Can you work these out from the model? Positions are in its coordinate system, mm. Face numbers are marked on the shaded views. A direction names the side the tool comes from. Give positions to 0.01 mm unless a question says otherwise; leave off trailing zeros. Write each loop counter-clockwise with the first axis right and the second up, starting at its lowest first coordinate (ties: lowest second). Pieces come first, ordered by that corner, then holes.
from build123d import *

# Parameters (mm, degrees)
SKETCH_1_R      = 1.5
EXTRUDE_1_DEPTH = 5


with BuildPart() as part:
    # 스케치1 → 보스-돌출1 (new body)
    with BuildSketch(Plane.XY):
        with BuildLine():
            Line((20.05, 5), (0, 5))
            ThreePointArc((0, 5), (-5, 0), (0, -5))
            Line((0, -5), (22, -5))
            Line((22, -5), (26.601353767, 1.956410875))
            Line((26.601353767, 1.956410875), (36.025134241, 5.963228766))
            Line((36.025134241, 5.963228766), (42.488975113, 3.018953392))
            Line((42.488975113, 3.018953392), (43.498164032, 3.018953392))
            Line((43.498164032, 3.018953392), (44.062133892, 4.253931713))
            Line((44.062133892, 4.253931713), (45.402427297, 4.470373499))
            Line((45.402427297, 4.470373499), (46.008680673, 5.685153438))
            Line((46.008680673, 5.685153438), (47.107948843, 5.685153438))
            Line((47.107948843, 5.685153438), (47.498446434, 6.712724429))
            Line((47.498446434, 6.712724429), (48.640951743, 6.712724429))
            Line((48.640951743, 6.712724429), (49.103035082, 7.757615508))
            Line((49.103035082, 7.757615508), (50.245112942, 7.726365831))
            Line((50.245112942, 7.726365831), (50.735603144, 8.758227131))
            Line((50.735603144, 8.758227131), (51.876398977, 8.69575116))
            Line((51.876398977, 8.69575116), (52.394929025, 9.713810574))
            Line((52.394929025, 9.713810574), (53.533589213, 9.620155058))
            Line((53.533589213, 9.620155058), (54.079771108, 10.623650806))
            Line((54.079771108, 10.623650806), (55.215443631, 10.498885825))
            Line((55.215443631, 10.498885825), (55.788868685, 11.487067026))
            Line((55.788868685, 11.487067026), (56.920703758, 11.331285936))
            Line((56.920703758, 11.331285936), (57.520942896, 12.303413169))
            Line((57.520942896, 12.303413169), (58.648093605, 12.116732536))
            Line((58.648093605, 12.116732536), (59.274697688, 13.072078391))
            Line((59.274697688, 13.072078391), (60.396320625, 12.854637901))
            Line((60.396320625, 12.854637901), (61.048820788, 13.792487525))
            Line((61.048820788, 13.792487525), (62.164076682, 13.544449883))
            Line((62.164076682, 13.544449883), (62.84198468, 14.464101515))
            Line((62.84198468, 14.464101515), (63.950039022, 14.185652318))
            Line((63.950039022, 14.185652318), (64.652847601, 15.086417815))
            Line((64.652847601, 15.086417815), (65.752871272, 14.777765417))
            Line((65.752871272, 14.777765417), (66.480054544, 15.658970767))
            Line((66.480054544, 15.658970767), (67.571224435, 15.320346122))
            Line((67.571224435, 15.320346122), (68.322238273, 16.181331949))
            Line((68.322238273, 16.181331949), (69.403737898, 15.812988438))
            Line((69.403737898, 15.812988438), (70.165521035, 16.650113087))
            Line((70.165521035, 16.650113087), (71.224188399, 16.249719983))
            Line((71.224188399, 16.249719983), (72.008283749, 17.065983242))
            Line((72.008283749, 17.065983242), (73.055761076, 16.637168043))
            Line((73.055761076, 16.637168043), (73.861597574, 17.431975419))
            Line((73.861597574, 17.431975419), (74.897121975, 16.975050435))
            Line((74.897121975, 16.975050435), (75.724112721, 17.74782306))
            Line((75.724112721, 17.74782306), (76.746930013, 17.263121075))
            Line((76.746930013, 17.263121075), (77.594472701, 18.013296132))
            Line((77.594472701, 18.013296132), (78.603837954, 17.501170159))
            Line((78.603837954, 17.501170159), (79.484104239, 18.229489901))
            Line((79.484104239, 18.229489901), (77.772918882, 22.391441928))
            Line((77.772918882, 22.391441928), (70.455863435, 25.724355994))
            Line((70.455863435, 25.724355994), (20.05, 5))
        make_face()
        with Locations((35.039512437, 8.36046215)):
            Circle(SKETCH_1_R, mode=Mode.SUBTRACT)
        Circle(SKETCH_1_R, mode=Mode.SUBTRACT)
        with Locations((22, 0)):
            Circle(SKETCH_1_R, mode=Mode.SUBTRACT)
        with Locations((67.410250422, 21.669681595)):
            Circle(SKETCH_1_R, mode=Mode.SUBTRACT)
    extrude(amount=EXTRUDE_1_DEPTH)


solid = part.part
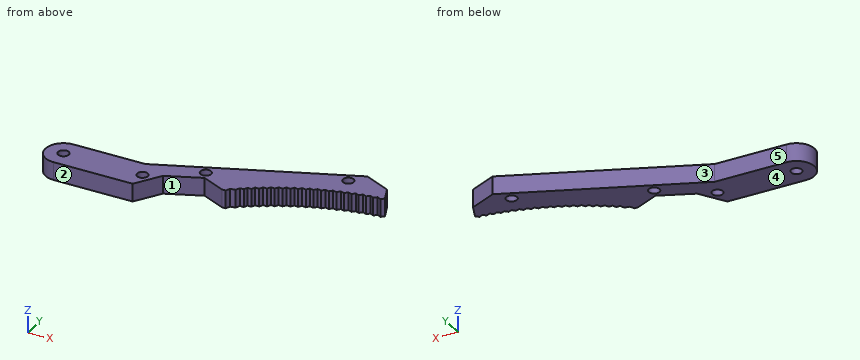
(1) Imagine slicing it at A-A, the plane y = 0. Write out the boundary of the cut face in (x, z).
Returned:
outline: (-5, 0) - (-1.5, 0) - (-1.5, 5) - (-5, 5) - close; (1.5, 0) - (20.5, 0) - (20.5, 5) - (1.5, 5) - close; (23.5, 0) - (25.31, 0) - (25.31, 5) - (23.5, 5) - close
(2) If I drill on L1, parallel to Y at x = 13.5, z = 2.55; L2, parallel to Y at x = 68, z = 1.1; L3, parallel to Y at x = 0, z = 2.7, over which ranges is the centre line in solid material (lowest first)?
Returned:
L1: y = -5 to 5
L2: y = 15.81 to 20.29, 23.05 to 24.71
L3: y = -5 to -1.5, 1.5 to 5
(3) Imagine slicing it at C-C, the plane x = 7. Write out the boundary of the cut face in (y, z), plus the area to 3 significant figures.
Returned:
outline: (-5, 0) - (5, 0) - (5, 5) - (-5, 5) - close
area: 50.0 mm2
(4) Imagine slicing it at B-B, the plane z = 2.05. Give the number of separate pieces and of enclosed holes in the cut face, plus the area to 3 significant figures.
Returned:
separate pieces: 1
enclosed holes: 4
area: 689 mm2
(5) If we mould it in two halves opening along X, with no side actions, what happens to the marked faces 1, 2 and 3? For each: +X half, -X half, draft (parallel to the pull), parting line (faces both ways), or undercut.
Returned:
face 1: undercut
face 2: draft
face 3: -X half
(6) For the marked faces 4 and 5, which set-ups out of +Z, -Z, +X, -X, +Y, -Y let a thin tool reach every point of the face, with its end or its side?
Returned:
face 4: -Z, +X, -X, +Y, -Y
face 5: +Z, -Z, -X, +Y
(7) Will these pins go through, and if not, where does the flat tip stop? P1, Ø1, axis at y = 8, z = 2.5, coming from the +X side; P2, Ø3.5, axis at x = 67.41, y = 21.67, coming from the -Z side; P3, Ø1, axis at x = 56, z = 2.5, coming from the +Y side; P4, Ø2.5, axis at x = 10, z = 1.5, coming from the +Y side.
Returned:
P1: stops at x = 50.61
P2: stops at z = 0
P3: stops at y = 19.99
P4: stops at y = 5
